Drawing for the job (mm, zero at the part's lowest x, y, z). A direction names the side the tool comes from. Give positions to 0.01 mm unless a question says otherwise; leave off trailing zeros. Loops run counter-clockwise (first coordinate to the right, second up) from the corner with the lowest first, then second, coordinate; pieces in that order, holes last. Notation, with made-up numbers: (84.5, 31) -> (104.5, 31) arc R22 cw to (104.5, 58) -> close; hole circle Ø4 at (11, -27). An arc over 180 degrees is marked (long way). Answer in a Markdown table with one row per item. Add a question column.
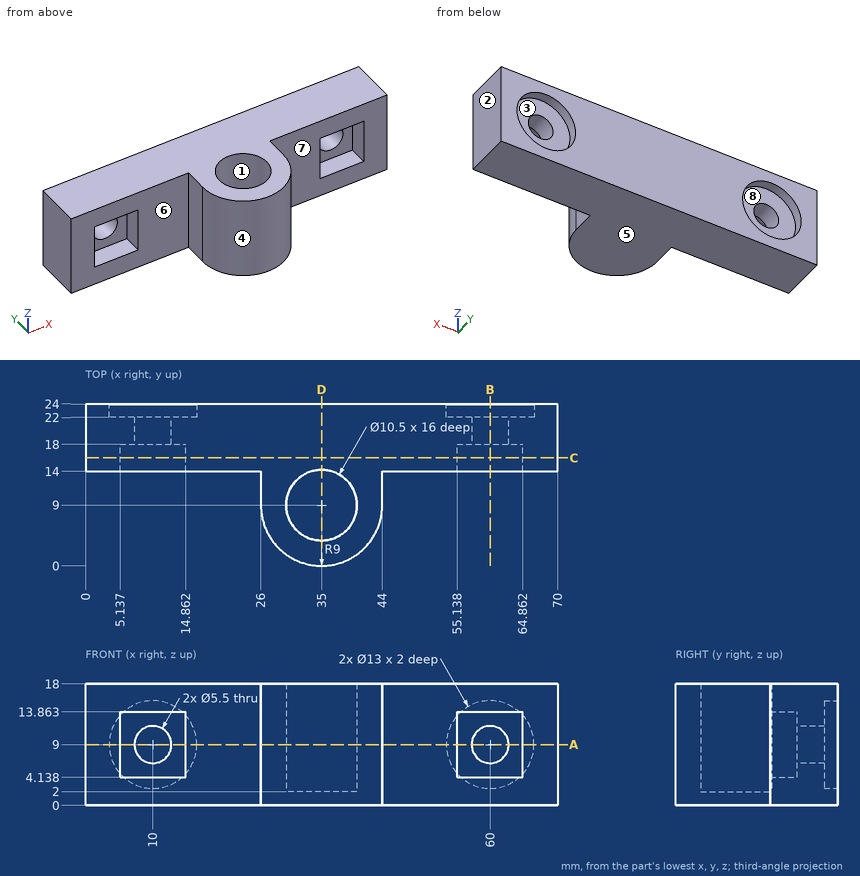
(1) Saw through at D-D, the plane x = 35. List the corners of the cut face in (y, z).
(2) Saw through at C-C, the plane y = 16. List the corners of the cut face in (x, z).
(3) Saw through at A-A, the plane z = 9. State how many separate pieces and enclosed holes the cut face has, then the cut area to 3 significant figures.
(4) 3-axis set-ups, long thin cutter, end or side, ignore diameter. For the marked faces 5, 6, 7 and 8: which of +Z, -Z, +X, -X, +Y, -Y reach the whole face in a straight line?
(5) Wall check: line 1 along Z through (x, y) = (10, 22.5); line 2 along X through (y, z) = (15.25, 6); line 3 along Z through (x, y) = (60, 19.4). Give the ranges that are in metal, low to high. Write a range as from..to.
(6) Two-plate mould, pull along X, no slides. Class the marked faces 1, 2, 3 and 4: released by +X, released by -X, zero draft, split by the parting line, or undercut.
(7) Flat gauge pins, fed straight in: pin 1 Ø6.5 at (x, z) = (60, 9) entering from +Y; pin 2 Ø8 at (y, z) = (9, 10) entering from +X; pin 3 Ø1.5 at (y, z) = (12.5, 14.5) entering from -X. Where does each tip first touch, or does it go through?
(8) Saw through at B-B, the plane x = 60. List the corners of the cut face in (y, z).
Worked answers:
| question | item | result |
|---|---|---|
| 1 | outline | (0, 0) -> (24, 0) -> (24, 18) -> (14.25, 18) -> (14.25, 2) -> (3.75, 2) -> (3.75, 18) -> (0, 18) -> close |
| 2 | outline | (0, 0) -> (70, 0) -> (70, 18) -> (0, 18) -> close; hole (5.14, 4.14) -> (14.86, 4.14) -> (14.86, 13.86) -> (5.14, 13.86) -> close; hole (55.14, 4.14) -> (64.86, 4.14) -> (64.86, 13.86) -> (55.14, 13.86) -> close |
| 3 | separate pieces | 3 |
| 3 | enclosed holes | 1 |
| 3 | area | 657 mm^2 |
| 4 | face 5 | -Z, +X, -X, +Y, -Y |
| 4 | face 6 | +Z, -Z, -X, -Y |
| 4 | face 7 | +Z, -Z, +X, -Y |
| 4 | face 8 | +Y |
| 5 | line 1 | 0..2.5, 15.5..18 |
| 5 | line 2 | 0..5.14, 14.86..55.14, 64.86..70 |
| 5 | line 3 | 0..6.25, 11.75..18 |
| 6 | face 1 | undercut |
| 6 | face 2 | released by +X |
| 6 | face 3 | undercut |
| 6 | face 4 | split by the parting line |
| 7 | pin 1 | y = 22 |
| 7 | pin 2 | x = 44 |
| 7 | pin 3 | x = 26 |
| 8 | outline | (14, 0) -> (24, 0) -> (24, 2.5) -> (22, 2.5) -> (22, 6.25) -> (18, 6.25) -> (18, 4.14) -> (14, 4.14) -> close; (14, 13.86) -> (18, 13.86) -> (18, 11.75) -> (22, 11.75) -> (22, 15.5) -> (24, 15.5) -> (24, 18) -> (14, 18) -> close |
